Geometry check sheet. Reference: the model listing, model coordinates, mm. Coordinates: 2 decimals unless noted, no trailing zeros. Loops run counter-clockwise (first coordinate to the right, second up) from the corner with the lowest first, then second, coordinate; pieces in that order, holes last. Notation, with made-up numbers: (9.5, -39) -> (52.5, -39) arc R29 ccw to (52.5, -17) -> close; hole circle Ø11 at (79.5, -38). An arc over 180 degrees is marked (long way). Answer as a JSON object with one key per item and string values.
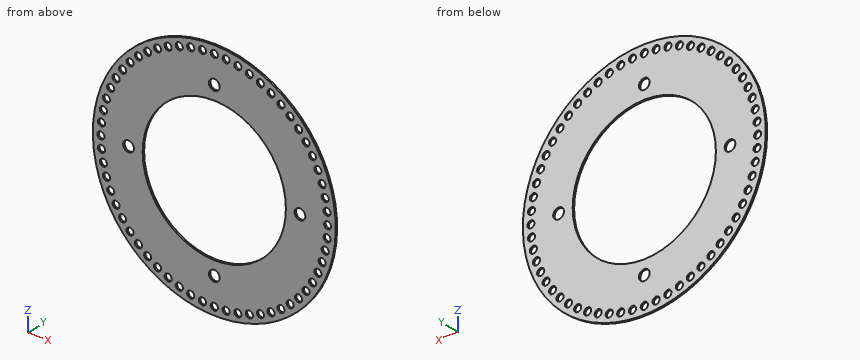
from build123d import *

# Parameters (mm, degrees)
SKETCH1_R           = 34
SKETCH1_R_2         = 20.05
BOSS_EXTRUDE1_DEPTH = 0.5
SKETCH2_R           = 1
CUT_EXTRUDE1_DEPTH  = 49.085860708
SKETCH3_R           = 1.5
CUT_EXTRUDE2_DEPTH  = 10


with BuildPart() as part:
    # Sketch1 → Boss-Extrude1 (new body)
    with BuildSketch(Plane(origin=(0, 0, 0), x_dir=(1, 0, 0), z_dir=(0, 1, 0))):
        with Locations(Location((0, 0, 0), (0, 0, 270))):
            Circle(SKETCH1_R)
        with Locations(Location((0, 0, 0), (0, 0, 270))):
            Circle(SKETCH1_R_2, mode=Mode.SUBTRACT)
    extrude(amount=BOSS_EXTRUDE1_DEPTH)

    # Sketch2 → Cut-Extrude1 (cut, through all)
    with BuildSketch(Plane(origin=(0, 0.5, 0), x_dir=(1, 0, 0), z_dir=(0, 1, 0))):
        with Locations(Location((0, 31.75, 0), (0, 0, 270))):
            Circle(SKETCH2_R)
        with Locations(Location((3.318778709, 31.576070178, 0), (0, 0, 270))):
            Circle(SKETCH2_R)
        with Locations(Location((6.601196183, 31.056186323, 0), (0, 0, 270))):
            Circle(SKETCH2_R)
        with Locations(Location((9.811289571, 30.196044392, 0), (0, 0, 270))):
            Circle(SKETCH2_R)
        with Locations(Location((12.913888418, 29.00506828, 0), (0, 0, 270))):
            Circle(SKETCH2_R)
        with Locations(Location((15.875, 27.49630657, 0), (0, 0, 270))):
            Circle(SKETCH2_R)
        with Locations(Location((18.66218176, 25.686289571, 0), (0, 0, 270))):
            Circle(SKETCH2_R)
        with Locations(Location((21.244896752, 23.594848209, 0), (0, 0, 270))):
            Circle(SKETCH2_R)
        with Locations(Location((23.594848209, 21.244896752, 0), (0, 0, 270))):
            Circle(SKETCH2_R)
        with Locations(Location((25.686289571, 18.66218176, 0), (0, 0, 270))):
            Circle(SKETCH2_R)
        with Locations(Location((27.49630657, 15.875, 0), (0, 0, 270))):
            Circle(SKETCH2_R)
        with Locations(Location((29.00506828, 12.913888418, 0), (0, 0, 270))):
            Circle(SKETCH2_R)
        with Locations(Location((30.196044392, 9.811289571, 0), (0, 0, 270))):
            Circle(SKETCH2_R)
        with Locations(Location((31.056186323, 6.601196183, 0), (0, 0, 270))):
            Circle(SKETCH2_R)
        with Locations(Location((31.576070178, 3.318778709, 0), (0, 0, 270))):
            Circle(SKETCH2_R)
        with Locations(Location((31.75, 0, 0), (0, 0, 270))):
            Circle(SKETCH2_R)
        with Locations(Location((31.576070178, -3.318778709, 0), (0, 0, 270))):
            Circle(SKETCH2_R)
        with Locations(Location((31.056186323, -6.601196183, 0), (0, 0, 270))):
            Circle(SKETCH2_R)
        with Locations(Location((30.196044392, -9.811289571, 0), (0, 0, 270))):
            Circle(SKETCH2_R)
        with Locations(Location((29.00506828, -12.913888418, 0), (0, 0, 270))):
            Circle(SKETCH2_R)
        with Locations(Location((27.49630657, -15.875, 0), (0, 0, 270))):
            Circle(SKETCH2_R)
        with Locations(Location((25.686289571, -18.66218176, 0), (0, 0, 270))):
            Circle(SKETCH2_R)
        with Locations(Location((23.594848209, -21.244896752, 0), (0, 0, 270))):
            Circle(SKETCH2_R)
        with Locations(Location((21.244896752, -23.594848209, 0), (0, 0, 270))):
            Circle(SKETCH2_R)
        with Locations(Location((18.66218176, -25.686289571, 0), (0, 0, 270))):
            Circle(SKETCH2_R)
        with Locations(Location((15.875, -27.49630657, 0), (0, 0, 270))):
            Circle(SKETCH2_R)
        with Locations(Location((12.913888418, -29.00506828, 0), (0, 0, 270))):
            Circle(SKETCH2_R)
        with Locations(Location((9.811289571, -30.196044392, 0), (0, 0, 270))):
            Circle(SKETCH2_R)
        with Locations(Location((6.601196183, -31.056186323, 0), (0, 0, 270))):
            Circle(SKETCH2_R)
        with Locations(Location((3.318778709, -31.576070178, 0), (0, 0, 270))):
            Circle(SKETCH2_R)
        with Locations(Location((0, -31.75, 0), (0, 0, 270))):
            Circle(SKETCH2_R)
        with Locations(Location((-3.318778709, -31.576070178, 0), (0, 0, 270))):
            Circle(SKETCH2_R)
        with Locations(Location((-6.601196183, -31.056186323, 0), (0, 0, 270))):
            Circle(SKETCH2_R)
        with Locations(Location((-9.811289571, -30.196044392, 0), (0, 0, 270))):
            Circle(SKETCH2_R)
        with Locations(Location((-12.913888418, -29.00506828, 0), (0, 0, 270))):
            Circle(SKETCH2_R)
        with Locations(Location((-15.875, -27.49630657, 0), (0, 0, 270))):
            Circle(SKETCH2_R)
        with Locations(Location((-18.66218176, -25.686289571, 0), (0, 0, 270))):
            Circle(SKETCH2_R)
        with Locations(Location((-21.244896752, -23.594848209, 0), (0, 0, 270))):
            Circle(SKETCH2_R)
        with Locations(Location((-23.594848209, -21.244896752, 0), (0, 0, 270))):
            Circle(SKETCH2_R)
        with Locations(Location((-25.686289571, -18.66218176, 0), (0, 0, 270))):
            Circle(SKETCH2_R)
        with Locations(Location((-27.49630657, -15.875, 0), (0, 0, 270))):
            Circle(SKETCH2_R)
        with Locations(Location((-29.00506828, -12.913888418, 0), (0, 0, 270))):
            Circle(SKETCH2_R)
        with Locations(Location((-30.196044392, -9.811289571, 0), (0, 0, 270))):
            Circle(SKETCH2_R)
        with Locations(Location((-31.056186323, -6.601196183, 0), (0, 0, 270))):
            Circle(SKETCH2_R)
        with Locations(Location((-31.576070178, -3.318778709, 0), (0, 0, 270))):
            Circle(SKETCH2_R)
        with Locations(Location((-31.75, 0, 0), (0, 0, 270))):
            Circle(SKETCH2_R)
        with Locations(Location((-31.576070178, 3.318778709, 0), (0, 0, 270))):
            Circle(SKETCH2_R)
        with Locations(Location((-31.056186323, 6.601196183, 0), (0, 0, 270))):
            Circle(SKETCH2_R)
        with Locations(Location((-30.196044392, 9.811289571, 0), (0, 0, 270))):
            Circle(SKETCH2_R)
        with Locations(Location((-29.00506828, 12.913888418, 0), (0, 0, 270))):
            Circle(SKETCH2_R)
        with Locations(Location((-27.49630657, 15.875, 0), (0, 0, 270))):
            Circle(SKETCH2_R)
        with Locations(Location((-25.686289571, 18.66218176, 0), (0, 0, 270))):
            Circle(SKETCH2_R)
        with Locations(Location((-23.594848209, 21.244896752, 0), (0, 0, 270))):
            Circle(SKETCH2_R)
        with Locations(Location((-21.244896752, 23.594848209, 0), (0, 0, 270))):
            Circle(SKETCH2_R)
        with Locations(Location((-18.66218176, 25.686289571, 0), (0, 0, 270))):
            Circle(SKETCH2_R)
        with Locations(Location((-15.875, 27.49630657, 0), (0, 0, 270))):
            Circle(SKETCH2_R)
        with Locations(Location((-12.913888418, 29.00506828, 0), (0, 0, 270))):
            Circle(SKETCH2_R)
        with Locations(Location((-9.811289571, 30.196044392, 0), (0, 0, 270))):
            Circle(SKETCH2_R)
        with Locations(Location((-6.601196183, 31.056186323, 0), (0, 0, 270))):
            Circle(SKETCH2_R)
        with Locations(Location((-3.318778709, 31.576070178, 0), (0, 0, 270))):
            Circle(SKETCH2_R)
    extrude(amount=-CUT_EXTRUDE1_DEPTH, mode=Mode.SUBTRACT)

    # Sketch3 → Cut-Extrude2 (cut)
    with BuildSketch(Plane(origin=(0, 0.5, 0), x_dir=(1, 0, 0), z_dir=(0, 1, 0))):
        with Locations(Location((0, 24, 0), (0, 0, 270))):
            Circle(SKETCH3_R)
        with Locations(Location((24, 0, 0), (0, 0, 270))):
            Circle(SKETCH3_R)
        with Locations(Location((0, -24, 0), (0, 0, 270))):
            Circle(SKETCH3_R)
        with Locations(Location((-24, 0, 0), (0, 0, 270))):
            Circle(SKETCH3_R)
    extrude(amount=-CUT_EXTRUDE2_DEPTH, mode=Mode.SUBTRACT)


solid = part.part
1. Section check B-B, the plane z = 10. Record the boundary of the cut face in (x, y).
Evaluation:
{"outline": "(-32.5, 0) -> (-31.18, 0) -> (-31.18, 0.5) -> (-32.5, 0.5) -> close; (-29.21, 0) -> (-17.38, 0) -> (-17.38, 0.5) -> (-29.21, 0.5) -> close; (17.38, 0) -> (29.21, 0) -> (29.21, 0.5) -> (17.38, 0.5) -> close; (31.18, 0) -> (32.5, 0) -> (32.5, 0.5) -> (31.18, 0.5) -> close"}
2. Depth check by flat-ended pin: P1, Ø1.8, axis at x = -27.5, z = 15.88, coming from the +Y side. Enter the tip coordinate at first touch or a pass-through.
Evaluation:
{"P1": "passes through"}
3. Thickness scan on probe 1 along Z at (x, y) = (-18, 0.4); probe 2 along X at (y, z) = (0.3, -21.5); probe 3 along Z at (x, y) = (-12.5, 0.45). Record the ranges inside material, lowest first. Write a range as from..to.
Evaluation:
{"probe 1": "z = -28.84..-26.44, -24.94..-8.83, 8.83..24.94, 26.44..28.84", "probe 2": "x = -26.34..-24.56, -22.63..22.63, 24.56..26.34", "probe 3": "z = -31.62..-29.92, -28.09..-15.68, 15.68..28.09, 29.92..31.62"}
4. Section check A-A, the plane z = -16. Record the boundary of the cut face in (x, y).
Evaluation:
{"outline": "(-30, 0) -> (-28.49, 0) -> (-28.49, 0.5) -> (-30, 0.5) -> close; (-26.5, 0) -> (-12.08, 0) -> (-12.08, 0.5) -> (-26.5, 0.5) -> close; (12.08, 0) -> (26.5, 0) -> (26.5, 0.5) -> (12.08, 0.5) -> close; (28.49, 0) -> (30, 0) -> (30, 0.5) -> (28.49, 0.5) -> close"}
5. Section check C-C, the plane y = 0.3. State how many separate pieces and enclosed holes the cut face has, then the cut area to 3 significant figures.
Evaluation:
{"separate pieces": "1", "enclosed holes": "65", "area": "2,150 mm^2"}
